Check sheet for the modelled part. Datum: model origin and axes. Units: mm. Face numbers are marked on the shaded views. Round coordinates to 2 decimals unless told otherwise and drop trailing zeros. Write each loop counter-clockwise with the first axis right and the second up, starting at its lowest first coordinate (ties: lowest second). Pieces come first, ordered by that corner, then holes. Notation, with made-up numbers: (-25, -22.75) -> (17, -22.75) arc R25 cw to (17, 12.25) -> close; hole circle Ø2 at (-11, 52.25). An arc over 180 degrees is marked (long way). One line per item, written item: value.
from build123d import *

# Parameters (mm, degrees)
SKETCH1_W               = 150
SKETCH1_H               = 45
BOSS_EXTRUDE1_DEPTH     = 260
CUT_EXTRUDE1_DEPTH      = 272.534988537
CUT_EXTRUDE1_DEPTH_BACK = 272.534988537
SKETCH2_W               = 144
SKETCH2_H               = 39
SKETCH3_W               = 96
SKETCH3_H               = 11.757854584
CUT_EXTRUDE2_DEPTH      = 526.862386942
SKETCH4_R               = 5
CUT_EXTRUDE3_DEPTH      = 302.008720804


with BuildPart() as part:
    # Sketch1 → Boss-Extrude1 (new, symmetric)
    with BuildSketch(Plane.XY):
        Rectangle(SKETCH1_W, SKETCH1_H)
    extrude(amount=BOSS_EXTRUDE1_DEPTH, both=True)

    # Sketch2 → Cut-Extrude1 (cut, two sides: drawn at the far end of the back side and taken through both)
    with BuildSketch(Plane.XY.offset(-CUT_EXTRUDE1_DEPTH_BACK)):
        Rectangle(SKETCH2_W, SKETCH2_H)
    extrude(amount=CUT_EXTRUDE1_DEPTH + CUT_EXTRUDE1_DEPTH_BACK, mode=Mode.SUBTRACT)

    # Sketch3 → Cut-Extrude2 (cut, through all)
    with BuildSketch(Plane.XY.offset(260)):
        with Locations((0, 22.5)):
            Rectangle(SKETCH3_W, SKETCH3_H)
    extrude(amount=-CUT_EXTRUDE2_DEPTH, mode=Mode.SUBTRACT)

    # Sketch4 → Cut-Extrude3 (cut, through all)
    with BuildSketch(Plane.ZY.offset(75)):
        with Locations((225, 0)):
            Circle(SKETCH4_R)
    extrude(amount=-CUT_EXTRUDE3_DEPTH, mode=Mode.SUBTRACT)


solid = part.part
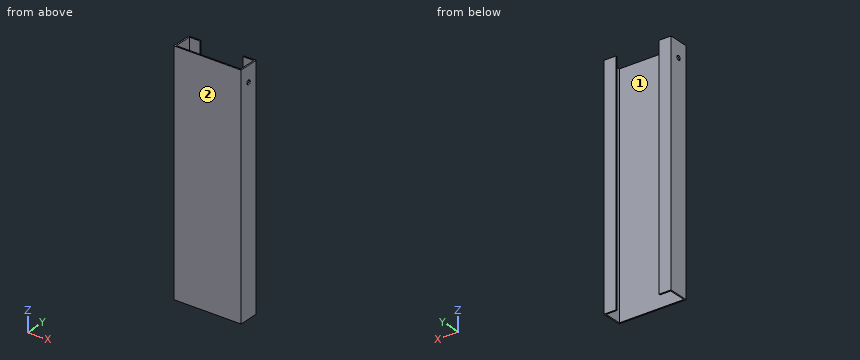
Item 1: Release check for a two-part mould opening along X. For the marked faces 1 and 2 record: pulls with the +X half, pulls with the -X half, needs draft (parallel to the pull), parting line crosses it, or undercut.
Result set:
face 1: undercut
face 2: needs draft
Item 2: Sectioned sample at C-C (z = 225). Enter the section's corners in (x, y), then the cut area to 3 significant figures.
Result set:
outline: (-75, -22.5) -> (75, -22.5) -> (75, -5) -> (72, -5) -> (72, -19.5) -> (-72, -19.5) -> (-72, -5) -> (-75, -5) -> close; (-75, 5) -> (-72, 5) -> (-72, 19.5) -> (-48, 19.5) -> (-48, 22.5) -> (-75, 22.5) -> close; (48, 19.5) -> (72, 19.5) -> (72, 5) -> (75, 5) -> (75, 22.5) -> (48, 22.5) -> close
area: 786 mm^2
Item 3: Material ranges on line 1 along X through (y, z) = (14.5, -164); line 2 along Y through (x, z) = (53, -35); line 3 along Y through (x, z) = (33, -26), recorded low to high.
Result set:
line 1: -75 to -72, 72 to 75
line 2: -22.5 to -19.5, 19.5 to 22.5
line 3: -22.5 to -19.5
Item 4: Sectioned sample at A-A (y = 0). Enter the section's corners in (x, z).
Result set:
outline: (-75, -260) -> (-72, -260) -> (-72, 220) -> (-75, 220) -> close; (-75, 230) -> (-72, 230) -> (-72, 260) -> (-75, 260) -> close; (72, -260) -> (75, -260) -> (75, 220) -> (72, 220) -> close; (72, 230) -> (75, 230) -> (75, 260) -> (72, 260) -> close
Item 5: Sectioned sample at D-D (z = -53). Enter the section's corners in (x, y), then the cut area to 3 significant figures.
Result set:
outline: (-75, -22.5) -> (75, -22.5) -> (75, 22.5) -> (48, 22.5) -> (48, 19.5) -> (72, 19.5) -> (72, -19.5) -> (-72, -19.5) -> (-72, 19.5) -> (-48, 19.5) -> (-48, 22.5) -> (-75, 22.5) -> close
area: 846 mm^2
Item 6: Sectioned sample at B-B (x = 64). Enter the section's corners in (y, z), then the cut area to 3 significant figures.
Result set:
outline: (-22.5, -260) -> (-19.5, -260) -> (-19.5, 260) -> (-22.5, 260) -> close; (19.5, -260) -> (22.5, -260) -> (22.5, 260) -> (19.5, 260) -> close
area: 3,120 mm^2
